Source: CAD feature listing. Evaluate the final solid. Frame: model axes, mm. A direction names the side the tool comes from. Coordinates: 2 decimals unless noted, no trailing zeros. Order: outer loops, then holes, each group sorted by start corner. A loop starts at its lowest first (then second) coordinate and runs counter-clockwise, first axis right, second up.
Autodesk Inventor part; units mm, degrees
ref_plane "YZ Plane" through (0, 0, 0) normal (1, 0, 0) x (0, 1, 0)
ref_plane "XZ Plane" through (0, 0, 0) normal (0, 1, 0) x (-1, 0, 0)
ref_plane "XY Plane" through (0, 0, 0) normal (0, 0, 1) x (1, 0, 0)
sketch "스케치1" plane through (0, 0, 0) normal (0, 1, 0) x (-1, 0, 0)
  line L0 (24.9446, -24.9446) -> (9.1304, -34.075)
  line L1 (9.1304, -34.075) -> (-9.1304, -34.075)
  line L2 (-9.1304, -34.075) -> (-24.9446, -24.9446)
  line L3 (-24.9446, -24.9446) -> (-34.075, -9.1304)
  line L4 (-34.075, -9.1304) -> (-34.075, 9.1304)
  line L5 (-34.075, 9.1304) -> (-24.9446, 24.9446)
  line L6 (-24.9446, 24.9446) -> (-9.1304, 34.075)
  line L7 (-9.1304, 34.075) -> (9.1304, 34.075)
  line L8 (9.1304, 34.075) -> (24.9446, 24.9446)
  line L9 (24.9446, 24.9446) -> (34.075, 9.1304)
  line L10 (34.075, 9.1304) -> (34.075, -9.1304)
  line L11 (34.075, -9.1304) -> (24.9446, -24.9446)
  line L12 (9.9878, -37.275) -> (-9.9878, -37.275)
  line L13 (-9.9878, -37.275) -> (-27.2872, -27.2872)
  line L14 (-27.2872, -27.2872) -> (-37.275, -9.9878)
  line L15 (-37.275, -9.9878) -> (-37.275, 9.9878)
  line L16 (-37.275, 9.9878) -> (-27.2872, 27.2872)
  line L17 (-27.2872, 27.2872) -> (-9.9878, 37.275)
  line L18 (-9.9878, 37.275) -> (9.9878, 37.275)
  line L19 (9.9878, 37.275) -> (27.2872, 27.2872)
  line L20 (27.2872, 27.2872) -> (37.275, 9.9878)
  line L21 (37.275, 9.9878) -> (37.275, -9.9878)
  line L22 (37.275, -9.9878) -> (27.2872, -27.2872)
  line L23 (27.2872, -27.2872) -> (9.9878, -37.275)
  point P0 (0, 0)
  point P1 (0, 0)
  point P2 (0, 0)
  dimension "d0" = 70.554
  dimension "d1" = 3.2
extrude "돌출1" add sketch "스케치1" along normal blind 3.7 contours L0 L1 L2 L3 L4 L5 L6 L7 L8 L9 L10 L11 | L12 L13 L14 L15 L16 L17 L18 L19 L20 L21 L22 L23
sketch "스케치2" plane through (0, 3.7, 0) normal (0, 1, 0) x (1, 0, 0)
  line L0 (-9.5591, 35.675) -> (9.5591, 35.675)
  line L1 (9.5591, 35.675) -> (26.1159, 26.1159)
  line L2 (26.1159, 26.1159) -> (35.675, 9.5591)
  line L3 (35.675, 9.5591) -> (35.675, -9.5591)
  line L4 (35.675, -9.5591) -> (26.1159, -26.1159)
  line L5 (26.1159, -26.1159) -> (9.5591, -35.675)
  line L6 (9.5591, -35.675) -> (-9.5591, -35.675)
  line L7 (-9.5591, -35.675) -> (-26.1159, -26.1159)
  line L8 (-26.1159, -26.1159) -> (-35.675, -9.5591)
  line L9 (-35.675, -9.5591) -> (-35.675, 9.5591)
  line L10 (-35.675, 9.5591) -> (-26.1159, 26.1159)
  line L11 (-26.1159, 26.1159) -> (-9.5591, 35.675)
  line L12 (9.9878, 37.275) -> (-9.9878, 37.275)
  point P0 (0, 0)
  point P1 (0, 0)
  point P2 (0, 35.675)
  dimension "d4" = 1.6
extrude "돌출2" cut sketch "스케치2" against normal blind 1.2
sketch "스케치3" plane through (0, 2.5, 0) normal (0, 1, 0) x (1, 0, 0)
  line L0 (-9.0232, 33.675) -> (9.0232, 33.675)
  line L1 (9.0232, 33.675) -> (24.6518, 24.6518)
  line L2 (24.6518, 24.6518) -> (33.675, 9.0232)
  line L3 (33.675, 9.0232) -> (33.675, -9.0232)
  line L4 (33.675, -9.0232) -> (24.6518, -24.6518)
  line L5 (24.6518, -24.6518) -> (9.0232, -33.675)
  line L6 (9.0232, -33.675) -> (-9.0232, -33.675)
  line L7 (-9.0232, -33.675) -> (-24.6518, -24.6518)
  line L8 (-24.6518, -24.6518) -> (-33.675, -9.0232)
  line L9 (-33.675, -9.0232) -> (-33.675, 9.0232)
  line L10 (-33.675, 9.0232) -> (-24.6518, 24.6518)
  line L11 (-24.6518, 24.6518) -> (-9.0232, 33.675)
  line L12 (-9.5591, 35.675) -> (9.5591, 35.675)
  point P0 (0, 0)
  point P1 (0, 0)
  dimension "d7" = 2
extrude "돌출3" add sketch "스케치3" along normal blind 0.6
fillet "모깎기1" radius 1.2 24 edges at (-18.6375, 3.7, 32.2811) (-32.2811, 3.7, 18.6375) (-37.275, 3.7, 0) (0, 3.7, 37.275) (18.6375, 3.7, 32.2811) (32.2811, 3.7, 18.6375) (37.275, 3.7, 0) (32.2811, 3.7, -18.6375) (18.6375, 3.7, -32.2811) (0, 3.7, -37.275) (-18.6375, 3.7, -32.2811) (-32.2811, 3.7, -18.6375) (-37.275, 0, 0) (-32.2811, 0, 18.6375) (-18.6375, 0, 32.2811) (0, 0, 37.275) (18.6375, 0, 32.2811) (32.2811, 0, 18.6375) (37.275, 0, 0) (32.2811, 0, -18.6375) (18.6375, 0, -32.2811) (0, 0, -37.275) (-18.6375, 0, -32.2811) (-32.2811, 0, -18.6375)
sketch "스케치10" plane through (0, 0, 0) normal (0, -1, 0) x (1, 0, 0)
  line L0 (10.3, 12.5) -> (15.3, 12.5)
  line L1 (15.3, 12.5) -> (15.3, -12.5)
  line L2 (15.3, -12.5) -> (10.3, -12.5)
  line L3 (10.3, -12.5) -> (10.3, 12.5)
  line L4 (10.3, 12.5) -> (15.3, -12.5) construction
  line L5 (15.3, 12.5) -> (10.3, -12.5) construction
  line L6 (0, 0) -> (0, -4.638)
  line L7 (-10.3, 12.5) -> (-15.3, 12.5)
  line L8 (-15.3, 12.5) -> (-15.3, -12.5)
  line L9 (-15.3, -12.5) -> (-10.3, -12.5)
  line L10 (-10.3, -12.5) -> (-10.3, 12.5)
  line L11 (-10.3, 12.5) -> (-15.3, -12.5) construction
  line L12 (-15.3, 12.5) -> (-10.3, -12.5) construction
  point P0 (12.8, 0)
  point P1 (-12.8, 0)
  dimension "d50" = 5
  dimension "d51" = 25
  dimension "d52" = 10.3
extrude "돌출7" add sketch "스케치10" along normal blind 15
sketch "스케치11" plane through (15.3, 0, 12.5) normal (1, 0, 0) x (0, 0, -1)
  circle A0 centre (7.5, -7.5) radius 1.25
  line L0 (2.8337, 0) -> (22.1663, 0)
  line L1 (12.5, 0) -> (12.5, -3.2899)
  circle A1 centre (17.5, -7.5) radius 1.25
  point P0 (12.5, 0)
  dimension "d55" = 2.5
  dimension "d56" = 7.5
  dimension "d57" = 5
extrude "돌출8" cut sketch "스케치11" against normal up to surface (30.6 mm away)
equation "\"d38\" = 55deg"
properties part number "OV-PAM_n_12_bottom"
Q1. Pin query (flat end, axial travel): P1, Ø3, axis at y = -7.5, z = -5, coming from the +X side; P2, Ø10, axis at x = -15, z = 18.5, coming from the -Y side; P3, Ø6, axis at y = -6, z = -2, coming from the -X side. Return the tip coordinate at first contact, or that it passes through.
Solutions:
P1: stops at x = 15.3
P2: stops at y = 0
P3: stops at x = -15.3
Q2. Section query A-A on z = -5. Give the number of separate pieces and of enclosed holes in the cut face, plus the area to 3 significant figures.
Solutions:
separate pieces: 3
enclosed holes: 0
area: 354 mm2
Q3. Section query C-C on y = -7.5. Output: boundary loops of the cut face in (x, z).
Solutions:
outline: (-15.3, -12.5) - (-10.3, -12.5) - (-10.3, -6.25) - (-15.3, -6.25) - close; (-15.3, -3.75) - (-10.3, -3.75) - (-10.3, 3.75) - (-15.3, 3.75) - close; (-15.3, 6.25) - (-10.3, 6.25) - (-10.3, 12.5) - (-15.3, 12.5) - close; (10.3, -12.5) - (15.3, -12.5) - (15.3, -6.25) - (10.3, -6.25) - close; (10.3, -3.75) - (15.3, -3.75) - (15.3, 3.75) - (10.3, 3.75) - close; (10.3, 6.25) - (15.3, 6.25) - (15.3, 12.5) - (10.3, 12.5) - close
Q4. Section query B-B on y = -2.5. Output: boundary loops of the cut face in (x, z).
Solutions:
outline: (-15.3, -12.5) - (-10.3, -12.5) - (-10.3, 12.5) - (-15.3, 12.5) - close; (10.3, -12.5) - (15.3, -12.5) - (15.3, 12.5) - (10.3, 12.5) - close
Q5. Set-up query: faces 1 (the flat face through (-15.3, -7, 0)), 2 (the flat face through (13, -7, 12.5)), 3 (the flat face through (10.3, -7, 0)), 4 (the flat face through (15.3, -7, 0)), 5 (the flat face through (18, 3.1, 30.8)). Return all of +Z, -Z, +X, -X, +Y, -Y with unobstructed straight access to the full face (end or side cutting, diameter ignored); none if empty.
Solutions:
face 1: +Z, -Z, -X, -Y
face 2: +Z, +X, -X, -Y
face 3: +Z, -Z, -Y
face 4: +Z, -Z, +X, -Y
face 5: +Y
Q6. Material intervals for line 1 along Y through (x, z) = (12.4, -5); line 2 along X through (y, z) = (-8.5, 8); line 3 along Y through (x, z) = (-30.5, -19), sorted ascending.
Solutions:
line 1: y = -15 to -8.75, -6.25 to 3.1
line 2: x = -15.3 to -10.3, 10.3 to 15.3
line 3: y = 0 to 3.7
